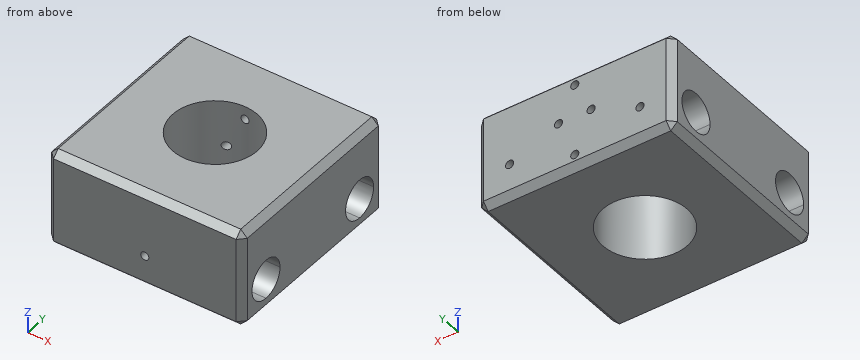
from build123d import *

# Parameters (mm, degrees)
SKETCH1_W           = 60
SKETCH1_H           = 60
SKETCH1_R           = 12.9
BOSS_EXTRUDE1_DEPTH = 30
CUT_EXTRUDE1_DEPTH  = 70
SKETCH3_R           = 1.25
CUT_EXTRUDE2_DEPTH  = 10
SKETCH4_R           = 1.25
CUT_EXTRUDE3_DEPTH  = 30
SKETCH5_R           = 1.25
CUT_EXTRUDE4_DEPTH  = 30
SKETCH6_R           = 1.25
CUT_EXTRUDE5_DEPTH  = 10
CHAMFER2_SIZE       = 2


with BuildPart() as part:
    # Sketch1 → Boss-Extrude1 (new body)
    with BuildSketch(Plane.XY):
        Rectangle(SKETCH1_W, SKETCH1_H)
        Circle(SKETCH1_R, mode=Mode.SUBTRACT)
    extrude(amount=BOSS_EXTRUDE1_DEPTH)

    # Sketch2 → Cut-Extrude1 (cut)
    with BuildSketch(Plane(origin=(30, 0, 0), x_dir=(0, 0, -1), z_dir=(1, 0, 0))):
        with BuildLine():
            ThreePointArc((-4, 20), (-5.757359313, 24.242640687), (-10, 26))
            Line((-10, 26), (-10, 14))
            ThreePointArc((-10, 14), (-5.757359313, 15.757359313), (-4, 20))
        make_face()
        with BuildLine():
            Line((-10, 14), (-10, 26))
            ThreePointArc((-10, 26), (-16, 20), (-10, 14))
        make_face()
        with BuildLine():
            ThreePointArc((-4, -20), (-5.757359313, -15.757359313), (-10, -14))
            Line((-10, -14), (-10, -26))
            ThreePointArc((-10, -26), (-5.757359313, -24.242640687), (-4, -20))
        make_face()
        with BuildLine():
            Line((-10, -26), (-10, -14))
            ThreePointArc((-10, -14), (-16, -20), (-10, -26))
        make_face()
    extrude(amount=-CUT_EXTRUDE1_DEPTH, mode=Mode.SUBTRACT)

    # Sketch3 → Cut-Extrude2 (cut)
    with BuildSketch(Plane(origin=(0, 30, 0), x_dir=(1, 0, 0), z_dir=(0, 1, 0))):
        with Locations(Location((-20, -10, 0), (0, 0, 270))):
            Circle(SKETCH3_R)
        with Locations(Location((20, -10, 0), (0, 0, 270))):
            Circle(SKETCH3_R)
    extrude(amount=-CUT_EXTRUDE2_DEPTH, mode=Mode.SUBTRACT)

    # Sketch4 → Cut-Extrude3 (cut)
    with BuildSketch(Plane(origin=(0, 30, 0), x_dir=(1, 0, 0), z_dir=(0, 1, 0))):
        with Locations(Location((-5, -16, 0), (0, 0, 270))):
            Circle(SKETCH4_R)
        with Locations(Location((5, -16, 0), (0, 0, 270))):
            Circle(SKETCH4_R)
    extrude(amount=-CUT_EXTRUDE3_DEPTH, mode=Mode.SUBTRACT)

    # Sketch5 → Cut-Extrude4 (cut)
    with BuildSketch(Plane(origin=(0, 30, 0), x_dir=(1, 0, 0), z_dir=(0, 1, 0))):
        with Locations(Location((0, -4, 0), (0, 0, 270))):
            Circle(SKETCH5_R)
        with Locations(Location((0, -26, 0), (0, 0, 270))):
            Circle(SKETCH5_R)
    extrude(amount=-CUT_EXTRUDE4_DEPTH, mode=Mode.SUBTRACT)

    # Sketch6 → Cut-Extrude5 (cut)
    with BuildSketch(Plane(origin=(0, -30, 0), x_dir=(-1, 0, 0), z_dir=(0, -1, 0))):
        with Locations(Location((0, -10, 0), (0, 0, 90))):
            Circle(SKETCH6_R)
    extrude(amount=-CUT_EXTRUDE5_DEPTH, mode=Mode.SUBTRACT)

    # Chamfer2
    chamfer2_edges = [part.edges().sort_by_distance(p)[0] for p in [
        (-30, 0, 30),
        (0, -30, 30),
        (30, 0, 30),
        (0, -30, 0),
        (-30, 0, 0),
        (0, 30, 0),
        (30, 0, 0),
        (0, 30, 30),
        (30, -30, 15),
        (-30, -30, 15),
        (-30, 30, 15),
        (30, 30, 15),
    ]]
    chamfer(chamfer2_edges, length=CHAMFER2_SIZE)


solid = part.part
Could you check a few things on this model? Use its own coordinates, in mm. Give positions to 0.01 mm unless a question says otherwise; leave off trailing zeros. Order: outer loops, then holes, each group sorted by start corner. A loop starts at its lowest first (then second) coordinate and runs counter-clockwise, first axis right, second up.
1. Suppose I cut it at A-A (y = 21). Write out the boundary of the cut face in (x, z), plus the area to 3 significant figures.
Answers below:
outline: (-30, 2) - (-28, 0) - (28, 0) - (30, 2) - (30, 4.08) - (1.25, 4.08) arc R1.25 cw (long way) to (-1.25, 4.08) - (-30, 4.08) - close; (-30, 15.92) - (-6.25, 15.92) arc R1.25 cw (long way) to (-3.75, 15.92) - (3.75, 15.92) arc R1.25 cw (long way) to (6.25, 15.92) - (30, 15.92) - (30, 28) - (28, 30) - (-28, 30) - (-30, 28) - close; hole circle Ø2.5 at (0, 26)
area: 1,070 mm2
2. Suppose I cut it at C-C (y = 0). Write out the boundary of the cut face in (x, z), plus the area to 3 significant figures.
Answers below:
outline: (-30, 2) - (-28, 0) - (-12.9, 0) - (-12.9, 30) - (-28, 30) - (-30, 28) - close; (12.9, 0) - (28, 0) - (30, 2) - (30, 28) - (28, 30) - (12.9, 30) - close
area: 1,020 mm2
3. Suppose I cut it at B-B (x = 20). Write out the boundary of the cut face in (y, z).
Answers below:
outline: (-30, 2) - (-28, 0) - (28, 0) - (30, 2) - (30, 8.75) - (25.87, 8.75) arc R6 cw (long way) to (25.87, 11.25) - (30, 11.25) - (30, 28) - (28, 30) - (-28, 30) - (-30, 28) - close; hole circle Ø12 at (-20, 10)
4. I need wall thicknesses on L1, parallel to X at y = 19, z = 16; L2, parallel to Z at x = 0, y = -27; L3, parallel to X at y = 27.05, z = 10. Which ranges of each line are inside material? Lowest first, please.
Answers below:
L1: x = -30 to -6.25, -3.75 to 3.75, 6.25 to 30
L2: z = 0 to 8.75, 11.25 to 30
L3: x = -30 to -21.25, -18.75 to 18.75, 21.25 to 30
5. For pin 1 (4 mm diameter, centred on x = 5, z = 16, fed in from +Y); pin 2 (12 mm diameter, centred on x = -2, y = 4, fed in from +Z); pin 3 (2 mm diameter, centred on x = 0, z = 26, fed in from +Y), each with a flat end and sliding along its axis, tell me the tip position at first contact or that it passes through.
Answers below:
pin 1: stops at y = 30
pin 2: passes through
pin 3: stops at y = -12.86
6. Suppose I cut it at D-D (z = 8). Write out the boundary of the cut face in (x, y), plus the area to 3 significant figures.
Answers below:
outline: (-30, -28) - (-28, -30) - (28, -30) - (30, -28) - (30, -25.66) - (-30, -25.66) - close; (-30, -14.34) - (30, -14.34) - (30, 14.34) - (-30, 14.34) - close; (-30, 25.66) - (30, 25.66) - (30, 28) - (28, 30) - (-28, 30) - (-30, 28) - close; hole circle Ø25.8 at (0, 0)
area: 1,710 mm2
